Source: CAD feature listing. Evaluate the final solid. Frame: model axes, mm. Face numbers are marked on the shaded views. A direction names the side the tool comes from. Give positions to 0.01 mm unless a question says otherwise; leave off trailing zeros. Loops run counter-clockwise (first coordinate to the right, second up) from the corner with the lowest first, then second, coordinate; pieces in that order, holes last. Notation, with made-up numbers: (-10, 63.25) - (24, 63.25) arc R31 cw to (24, 93.25) - close; hole circle Ø6 at (49, -38.5). An arc over 180 degrees is marked (long way). Put each result on its own line as item: value.
```python
from build123d import *

# Parameters (mm, degrees)
EXTRUDE_1_DEPTH = 15
EXTRUDE_4_DEPTH = 15


with BuildPart() as part:
    # 草图1 → 凸台-拉伸1 (new body)
    with BuildSketch(Plane(origin=(0, 0, 0), x_dir=(1, 0, 0), z_dir=(0, 1, 0))):
        Polygon((-20.642691415, 18.026682135), (-20.642691415, -24.110208817), (20.357308585, -24.110208817), (20.357308585, 18.026682135), (24.357308585, 18.026682135), (24.357308585, -28.110208817), (-24.642691415, -28.110208817), (-24.642691415, 18.026682135), align=None)
    extrude(amount=EXTRUDE_1_DEPTH)

    # 草图3 → 凸台-拉伸4 (add)
    with BuildSketch(Plane.XZ):
        with BuildLine():
            Line((-24.642691415, 28.110208817), (-24.642691415, 32.110208817))
            Line((-24.642691415, 32.110208817), (-17.486324867, 32.110208817))
            ThreePointArc((-17.486324867, 32.110208817), (-18.930816259, 30.370057744), (-19.018929604, 28.110208817))
            Line((-19.018929604, 28.110208817), (-24.642691415, 28.110208817))
        make_face()
        with BuildLine():
            Line((-13.839915778, 32.110208817), (-7.445467053, 32.110208817))
            ThreePointArc((-7.445467053, 32.110208817), (-8.905871866, 30.375773254), (-8.996793382, 28.110208817))
            Line((-8.996793382, 28.110208817), (-12.288589449, 28.110208817))
            ThreePointArc((-12.288589449, 28.110208817), (-12.379510964, 30.375773254), (-13.839915778, 32.110208817))
        make_face()
        with BuildLine():
            Line((-3.839915778, 32.110208817), (3.554532947, 32.110208817))
            ThreePointArc((3.554532947, 32.110208817), (2.094128134, 30.375773254), (2.003206618, 28.110208817))
            Line((2.003206618, 28.110208817), (-2.288589449, 28.110208817))
            ThreePointArc((-2.288589449, 28.110208817), (-2.379510964, 30.375773254), (-3.839915778, 32.110208817))
        make_face()
        with BuildLine():
            Line((7.160084222, 32.110208817), (13.554532947, 32.110208817))
            ThreePointArc((13.554532947, 32.110208817), (12.094128134, 30.375773254), (12.003206618, 28.110208817))
            Line((12.003206618, 28.110208817), (8.70892166, 28.101898452))
            ThreePointArc((8.70892166, 28.101898452), (8.622054937, 30.371728239), (7.160084222, 32.110208817))
        make_face()
        with BuildLine():
            Line((17.160084222, 32.110208817), (24.357308585, 32.110208817))
            Line((24.357308585, 32.110208817), (24.357308585, 28.110208817))
            Line((24.357308585, 28.110208817), (18.711410551, 28.110208817))
            ThreePointArc((18.711410551, 28.110208817), (18.620489036, 30.375773254), (17.160084222, 32.110208817))
        make_face()
    extrude(amount=-EXTRUDE_4_DEPTH)


solid = part.part
```
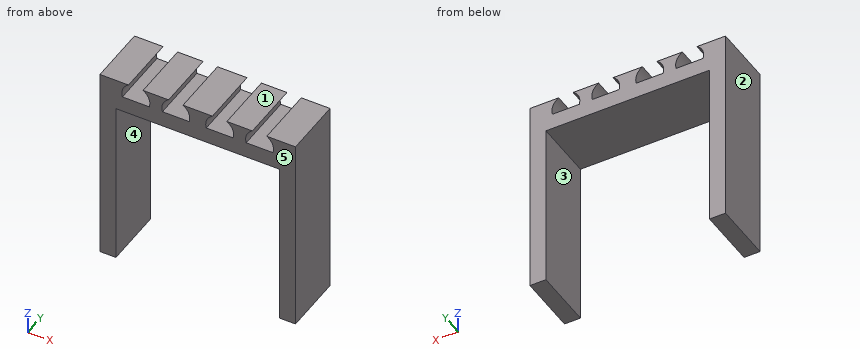
1) Material intervals for line 1 along X through (y, z) = (14.5, -13); line 2 along Z through (x, y) = (-1, 5.75); line 3 along Z through (x, y) = (-17, 3), sorted ascending. Write a range as [from, to].
Check result:
line 1: [-24.64, -20.64], [20.36, 24.36]
line 2: [24.11, 32.11]
line 3: [24.11, 28.11]
2) Section query B-B, the plane y = 11.75. Output: boundary loops of the cut face in (x, z).
Check result:
outline: (-24.64, -18.03) - (-20.64, -18.03) - (-20.64, 24.11) - (20.36, 24.11) - (20.36, -18.03) - (24.36, -18.03) - (24.36, 32.11) - (17.16, 32.11) arc R3.5 cw to (18.71, 28.11) - (12, 28.11) arc R3.5 cw to (13.55, 32.11) - (7.16, 32.11) arc R3.5 cw to (8.71, 28.11) - (2, 28.11) arc R3.5 cw to (3.55, 32.11) - (-3.84, 32.11) arc R3.5 cw to (-2.29, 28.11) - (-9, 28.11) arc R3.5 cw to (-7.45, 32.11) - (-13.84, 32.11) arc R3.5 cw to (-12.29, 28.11) - (-19.02, 28.11) arc R3.52 cw to (-17.49, 32.11) - (-24.64, 32.11) - close
3) Access query for the marked faces 4 and 5. Directions: +Z, -Z, +X, -X, +Y, -Y. A direction counts if a zero-diameter tool reaches every point of the face in a straight line with its end or side. Return the directions, or none.
Check result:
face 4: -Z, +Y, -Y
face 5: +Z, -Z, +X, -X, -Y
4) Pin query (flat end, axial travel): P1, Ø1, axis at x = -15.5, y = 2.5, coming from the +Z side; P2, Ø3, axis at x = -16, y = 7, coming from the -Z side. Return the tip coordinate at first contact, or that it passes through.
Check result:
P1: z = 28.11
P2: z = 24.11
5) Section query A-A, the plane z = -6. Output: boundary loops of the cut face in (x, y).
Check result:
outline: (-24.64, 0) - (-20.64, 0) - (-20.64, 15) - (-24.64, 15) - close; (20.36, 0) - (24.36, 0) - (24.36, 15) - (20.36, 15) - close
6) Mould query, pull axis X, two halves, no side actions, for the marked faces 1, 2 and 3. Classes: pulls with the +X half, pulls with the -X half, needs draft (parallel to the pull), parting line crosses it, or undercut.
Check result:
face 1: needs draft
face 2: pulls with the -X half
face 3: undercut
